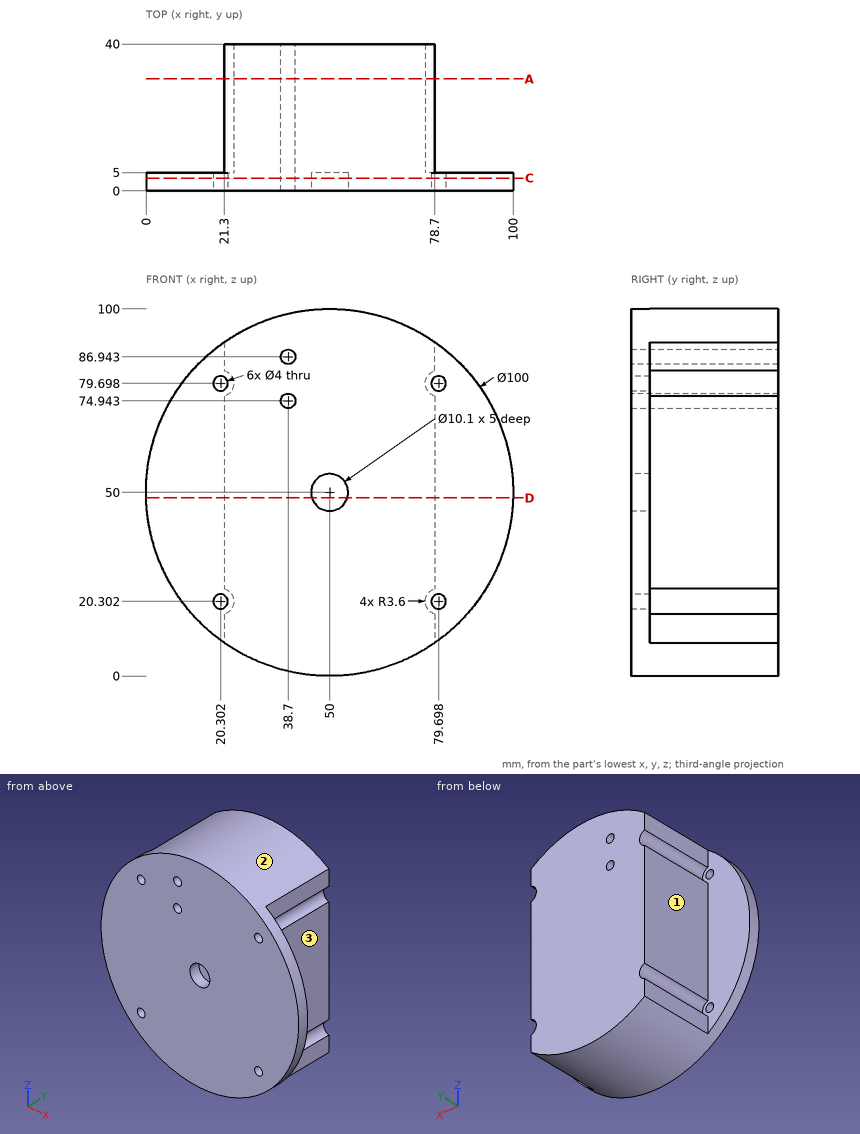
For this review, use the dimensioned drawing (mm, ordinates from the lowest corner) and the shaded views. A direction names the side the tool comes from. Give positions to 0.01 mm unless a question says otherwise; leave off trailing zeros. Order: outer loops, then holes, each group sorted by start corner. A loop starts at its lowest first (then second) coordinate and runs counter-clockwise, first axis right, second up. Notation, with made-up numbers: (-22, 23) - (-6, 23) arc R14 ccw to (-6, 38) - close; hole circle Ø1 at (73, 19.25). An arc over 180 degrees is marked (long way). Use a Markdown table: item, result. Add a question column.
(1) Clearance check with flat-ended pins moving along their axes: P1, Ø4.5, axis at x = 79.7, z = 20.3, coming from the +Y side; P2, Ø17.5, axis at y = 17, z = 37, coming from the +X side; P3, Ø8.5, axis at y = 26, z = 12, coming from the -X side; P4, Ø2.5, axis at x = 79.7, z = 79.7, coming from the -Y side. State where each tip first meets the part, or that it passes through.
(2) Machinability: for the marked faces 1, 2 and 3, which of the approach directions +Z, -Z, +X, -X, +Y, -Y give a long, thin tool a straight path to every point of the face, cutting with its end or side? Answer none if there is none.
(3) Wall thickness on probe 1 along X at (y, z) = (29, 31); probe 2 along Y at (x, z) = (80.5, 59); probe 3 along Z at (x, y) = (50, 8): over which ranges is each line inside the solid? List them lowest first. Write a range as [from, to].
(4) Add section A-A on y = 30.5. Give the boundary of the cut face in (x, z), then the cut area to 3 significant figures.
(5) Add section C-C on y = 3.5. Give the boundary of the cut face in (x, z).
(6) Add section D-D on z = 48.5. Give the boundary of the cut face in (x, y), then the cut area to 3 significant figures.
Report:
| question | item | result |
|---|---|---|
| 1 | P1 | stops at y = 5 |
| 1 | P2 | stops at x = 78.7 |
| 1 | P3 | stops at x = 21.3 |
| 1 | P4 | passes through |
| 2 | face 1 | +Z, -Z, -X, +Y |
| 2 | face 2 | +Y, -Y |
| 2 | face 3 | +Z, -Z, +X, +Y |
| 3 | probe 1 | x = [21.3, 78.7] |
| 3 | probe 2 | y = [0, 5] |
| 3 | probe 3 | z = [0, 100] |
| 4 | outline | (21.3, 9.06) arc R50 ccw to (78.7, 9.06) - (78.7, 16.84) arc R3.6 cw to (78.7, 23.76) - (78.7, 76.24) arc R3.6 cw to (78.7, 83.16) - (78.7, 90.94) arc R50 ccw to (21.3, 90.94) - (21.3, 83.16) arc R3.6 cw to (21.3, 76.24) - (21.3, 23.76) arc R3.6 cw to (21.3, 16.84) - close; hole circle Ø4 at (38.7, 74.94); hole circle Ø4 at (38.7, 86.94) |
| 4 | area | 5,330 mm² |
| 5 | outline | circle Ø100 at (50, 50); hole circle Ø4 at (20.3, 20.3); hole circle Ø4 at (20.3, 79.7); hole circle Ø4 at (38.7, 74.94); hole circle Ø4 at (38.7, 86.94); hole circle Ø10.1 at (50, 50); hole circle Ø4 at (79.7, 20.3); hole circle Ø4 at (79.7, 79.7) |
| 6 | outline | (0.02, 0) - (45.18, 0) - (45.18, 5) - (54.82, 5) - (54.82, 0) - (99.98, 0) - (99.98, 5) - (78.7, 5) - (78.7, 40) - (21.3, 40) - (21.3, 5) - (0.02, 5) - close |
| 6 | area | 2,460 mm² |
